from build123d import *

# Parameters (mm, degrees)
SKETCH5_W               = 241
SKETCH5_H               = 130
BOSS_EXTRUDE2_DEPTH     = 20
SKETCH6_W               = 20
SKETCH6_H               = 90
BOSS_EXTRUDE3_DEPTH     = 100
CUT_EXTRUDE1_DEPTH      = 269.897750084
CUT_EXTRUDE1_DEPTH_BACK = 269.897750084
SKETCH8_R               = 24.784776311
SKETCH9_R               = 15.5
CUT_EXTRUDE2_DEPTH      = 10
SKETCH10_R              = 1
CUT_EXTRUDE3_DEPTH      = 20


with BuildPart() as part:
    # Sketch5 → Boss-Extrude2 (new body)
    with BuildSketch(Plane(origin=(0, 0, 0), x_dir=(1, 0, 0), z_dir=(0, 1, 0))):
        Rectangle(SKETCH5_W, SKETCH5_H)
    extrude(amount=-BOSS_EXTRUDE2_DEPTH)

    # Sketch6 → Boss-Extrude3 (add)
    with BuildSketch(Plane(origin=(0, 0, 0), x_dir=(1, 0, 0), z_dir=(0, 1, 0))):
        with Locations((110.5, 0)):
            Rectangle(SKETCH6_W, SKETCH6_H)
        with Locations((-110.5, 0)):
            Rectangle(SKETCH6_W, SKETCH6_H)
    extrude(amount=BOSS_EXTRUDE3_DEPTH)

    # Sketch8 → Cut-Extrude1 (cut, two sides: drawn at the far end of the back side and taken through both)
    with BuildSketch(Plane(origin=(120.5, 0, 0), x_dir=(0, 0, -1), z_dir=(1, 0, 0)).offset(-CUT_EXTRUDE1_DEPTH_BACK)):
        with Locations((0, 50)):
            Circle(SKETCH8_R)
    extrude(amount=CUT_EXTRUDE1_DEPTH + CUT_EXTRUDE1_DEPTH_BACK, mode=Mode.SUBTRACT)

    # Sketch9 → Cut-Extrude2 (cut)
    with BuildSketch(Plane.XZ.offset(20)):
        with Locations(Location((0, 0, 0), (0, 0, 270))):
            Circle(SKETCH9_R)
    extrude(amount=-CUT_EXTRUDE2_DEPTH, mode=Mode.SUBTRACT)

    # Sketch10 → Cut-Extrude3 (cut)
    with BuildSketch(Plane(origin=(120.5, 0, 0), x_dir=(0, 0, -1), z_dir=(1, 0, 0))):
        with Locations((0, 81)):
            Circle(SKETCH10_R)
        with Locations((-31, 50)):
            Circle(SKETCH10_R)
        with Locations((31, 50)):
            Circle(SKETCH10_R)
        with Locations((0, 19)):
            Circle(SKETCH10_R)
    extrude(amount=-CUT_EXTRUDE3_DEPTH, mode=Mode.SUBTRACT)


solid = part.part
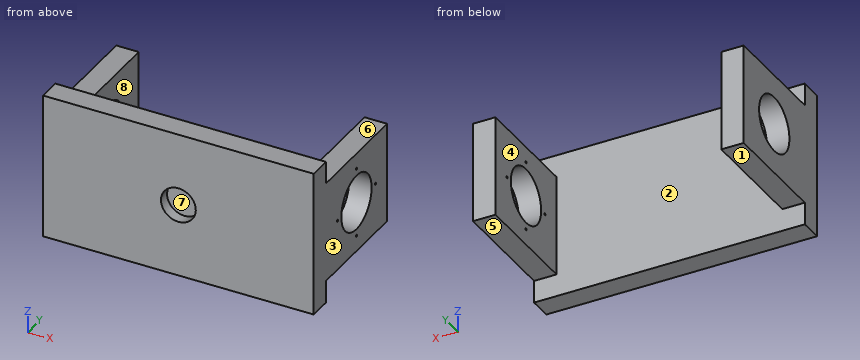
Work out the finished part from the listing and answer in its coordinate system (mm). Face numbers are marked on the shaded views. A direction names the side the tool comes from. Give positions to 0.01 mm unless a question says otherwise; leave off trailing zeros. Order: outer loops, then holes, each group sorted by start corner. A loop starts at its lowest first (then second) coordinate and runs counter-clockwise, first axis right, second up. Notation, with made-up numbers: (-13, 14.25) - (7, 14.25) arc R18 ccw to (7, 46.25) - close; hole circle Ø3 at (23.25, 63.25). An arc over 180 degrees is marked (long way). Answer as CSV lines item,"result". Start each with the question number.
Q1. Given pin 1 Ø22 at (x, y) = (-107.5, 49) entering from +Z; pin 2 Ø1.8 at (y, z) = (50, -31) entering from +X; pin 3 Ø6 at (x, z) = (-76, -46) entering from +Y, each flat-ended and moving along its own axis, determine where each tip first touches the part or whether it passes through.
Q2. The part is cut by section D-D (y = 59). Write down the section's boundary in (x, z), then the cut area to 3 significant figures.
Q3. The part is cut by section C-C (z = -40). Write down the section's boundary in (x, y).
Q4. The mould has two halves that part along X. Classify the marked faces 1, 2, 3 and 4: +X half, -X half, draft (parallel to the pull), parting line (faces both ways), or undercut.
Q5. For the marked faces 5, 6, 7 and 8, determine the directions among +Z, -Z, +X, -X, +Y, -Y from which every point of the face is accessible in a straight line to the end or side of a thin tool.
Q6. The part is cut by section A-A (y = 71). Write down the section's boundary in (x, z), then the cut area to 3 significant figures.
Q7. Find the intervals of material crossed by L1, parallel to Y at x = 110.5, z = 0; L2, parallel to X at y = -17, z = 0; L3, parallel to X at y = 2.5, z = 17.5, in increasing order. Write a range as [from, to].
Q8. The part is cut by section B-B (z = -4). Write down the section's boundary in (x, y).
Check result:
1,pin 1,"stops at z = 45"
1,pin 2,"stops at x = -100.5"
1,pin 3,"stops at y = 0"
2,outline,"(-120.5, -45) - (-100.5, -45) - (-100.5, -23.09) - (-120.5, -23.09) - close; (-120.5, 23.09) - (-100.5, 23.09) - (-100.5, 45) - (-120.5, 45) - close; (100.5, -45) - (120.5, -45) - (120.5, -23.09) - (100.5, -23.09) - close; (100.5, 23.09) - (120.5, 23.09) - (120.5, 45) - (100.5, 45) - close"
2,area,"1,750 mm²"
3,outline,"(-120.5, -20) - (120.5, -20) - (120.5, 100) - (100.5, 100) - (100.5, 0) - (-100.5, 0) - (-100.5, 100) - (-120.5, 100) - close"
4,face 1,"draft"
4,face 2,"undercut"
4,face 3,"+X half"
4,face 4,"undercut"
5,face 5,"-Z, +X, -X, +Y"
5,face 6,"+Z, +X, -X, +Y"
5,face 7,"-Y"
5,face 8,"+Z, -Z, +Y"
6,outline,"(-120.5, -45) - (-100.5, -45) - (-100.5, -13.16) - (-120.5, -13.16) - close; (-120.5, 13.16) - (-100.5, 13.16) - (-100.5, 45) - (-120.5, 45) - close; (100.5, -45) - (120.5, -45) - (120.5, -13.16) - (100.5, -13.16) - close; (100.5, 13.16) - (120.5, 13.16) - (120.5, 45) - (100.5, 45) - close"
6,area,"2,550 mm²"
7,L1,"y = [-20, 18], [20, 25.22], [74.78, 80], [82, 100]"
7,L2,"x = [-120.5, -15.5], [15.5, 120.5]"
7,L3,"x = [-120.5, -100.5], [100.5, 120.5]"
8,outline,"(-120.5, -20) - (-14.97, -20) - (-14.97, -10) - (14.97, -10) - (14.97, -20) - (120.5, -20) - (120.5, 25.54) - (100.5, 25.54) - (100.5, 0) - (-100.5, 0) - (-100.5, 25.54) - (-120.5, 25.54) - close; (-120.5, 74.46) - (-100.5, 74.46) - (-100.5, 100) - (-120.5, 100) - close; (100.5, 74.46) - (120.5, 74.46) - (120.5, 100) - (100.5, 100) - close"
